For this review, take the finished solid that the model builds, in its own axes (mm). Face numbers are marked on the shaded views. A direction names the side the tool comes from. Coordinates: 2 decimals unless noted, no trailing zeros. Loops run counter-clockwise (first coordinate to the right, second up) from the corner with the lowest first, then second, coordinate; pieces in that order, holes last. Notation, with made-up numbers: (24, -28) - (55, -28) arc R31 ccw to (55, 6) - close; hole circle Ø2 at (84, 68.25). An arc over 180 degrees is marked (long way). Answer as a JSON object with one key per item and string values. Group by question number.
Item 1: Clearance check with flat-ended pins moving along their axes: pin 1 (0.5 mm diameter, centred on y = 1, z = 3, fed in from +X); pin 2 (0.5 mm diameter, centred on y = 2, z = -3, fed in from -X); pin 3 (0.9 mm diameter, centred on x = 5, y = 1, fed in from +Z). State where each tip first meets the part, or that it passes through.
Item 2: Tool access review of the marked faces 4, 5, 6 and 7: name each direction out of +Z, -Z, +X, -X, +Y, -Y from which nothing blocks a thin tool from reaching the whole face with its end or side.
Item 3: We need section C-C (y = 0.7). Give the boundary of the cut face in (x, z), then the cut area to 3 significant figures.
Item 4: We need section A-A (z = 1.5). Give the boundary of the cut face in (x, y), then the cut area to 3 significant figures.
Item 5: We need section D-D (x = 4.25). Give the boundary of the cut face in (y, z), then the cut area to 3 significant figures.
Item 6: We need section B-B (x = 1.75). Give the boundary of the cut face in (y, z), then the cut area to 3 significant figures.
Item 7: Mouldability with a two-part tool opening along Z and no side actions: class the marked faces 1, 2 and 3 as released by +Z, released by -Z, zero draft, split by the parting line, or undercut.
Item 8: To check wall thickness, follow line 1 (Z direction, x = 0.25, y = 1.45); line 2 (X direction, y = 2.3, z = 2); line 3 (Z direction, x = 3.75, y = 0.6). State the ranges of each line that lie inside material, in increasing order.
from build123d import *

# Parameters (mm, degrees)
SKETCH1_W           = 7
SKETCH1_H           = 7
BOSS_EXTRUDE1_DEPTH = 3
SKETCH4_W           = 3
SKETCH4_H           = 5
BOSS_EXTRUDE2_DEPTH = 3
SKETCH5_W           = 6
SKETCH5_H           = 6
CUT_EXTRUDE1_DEPTH  = 10


with BuildPart() as part:
    # Sketch1 → Boss-Extrude1 (new body)
    with BuildSketch(Plane(origin=(0, 0, 0), x_dir=(1, 0, 0), z_dir=(0, 1, 0))):
        Rectangle(SKETCH1_W, SKETCH1_H)
    extrude(amount=BOSS_EXTRUDE1_DEPTH)

    # Sketch4 → Boss-Extrude2 (add)
    with BuildSketch(Plane(origin=(0, 3, 0), x_dir=(1, 0, 0), z_dir=(0, 1, 0))):
        with Locations((-5, 0)):
            Rectangle(SKETCH4_W, SKETCH4_H)
        with Locations((5, 0)):
            Rectangle(SKETCH4_W, SKETCH4_H)
    extrude(amount=-BOSS_EXTRUDE2_DEPTH)

    # Sketch5 → Cut-Extrude1 (cut)
    with BuildSketch(Plane(origin=(0, 3, 0), x_dir=(1, 0, 0), z_dir=(0, 1, 0))):
        Rectangle(SKETCH5_W, SKETCH5_H)
    extrude(amount=-CUT_EXTRUDE1_DEPTH, mode=Mode.SUBTRACT)


solid = part.part
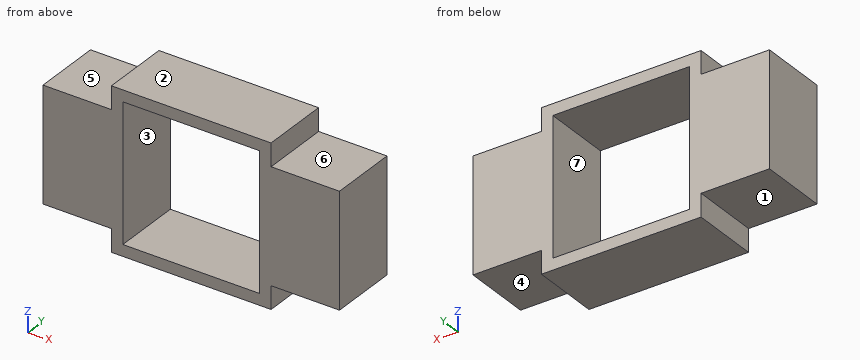
Check sheet entries:
{
 "1": {"pin 1": "stops at x = 3.5", "pin 2": "stops at x = -3.5", "pin 3": "stops at z = 2.5"},
 "2": {"face 4": "-Z, +X, +Y, -Y", "face 5": "+Z, -X, +Y, -Y", "face 6": "+Z, +X, +Y, -Y", "face 7": "+Y, -Y"},
 "3": {"outline": "(-6.5, -2.5) - (-3.5, -2.5) - (-3.5, -3.5) - (3.5, -3.5) - (3.5, -2.5) - (6.5, -2.5) - (6.5, 2.5) - (3.5, 2.5) - (3.5, 3.5) - (-3.5, 3.5) - (-3.5, 2.5) - (-6.5, 2.5) - close; hole (-3, -3) - (3, -3) - (3, 3) - (-3, 3) - close", "area": "43.0 mm2"},
 "4": {"outline": "(-6.5, 0) - (-3, 0) - (-3, 3) - (-6.5, 3) - close; (3, 0) - (6.5, 0) - (6.5, 3) - (3, 3) - close", "area": "21.0 mm2"},
 "5": {"outline": "(0, -2.5) - (3, -2.5) - (3, 2.5) - (0, 2.5) - close", "area": "15.0 mm2"},
 "6": {"outline": "(0, -3.5) - (3, -3.5) - (3, -3) - (0, -3) - close; (0, 3) - (3, 3) - (3, 3.5) - (0, 3.5) - close", "area": "3.00 mm2"},
 "7": {"face 1": "released by -Z", "face 2": "released by +Z", "face 3": "undercut"},
 "8": {"line 1": "z = -3.5 to -3, 3 to 3.5", "line 2": "x = -6.5 to -3, 3 to 6.5", "line 3": "z = -2.5 to 2.5"}
}
